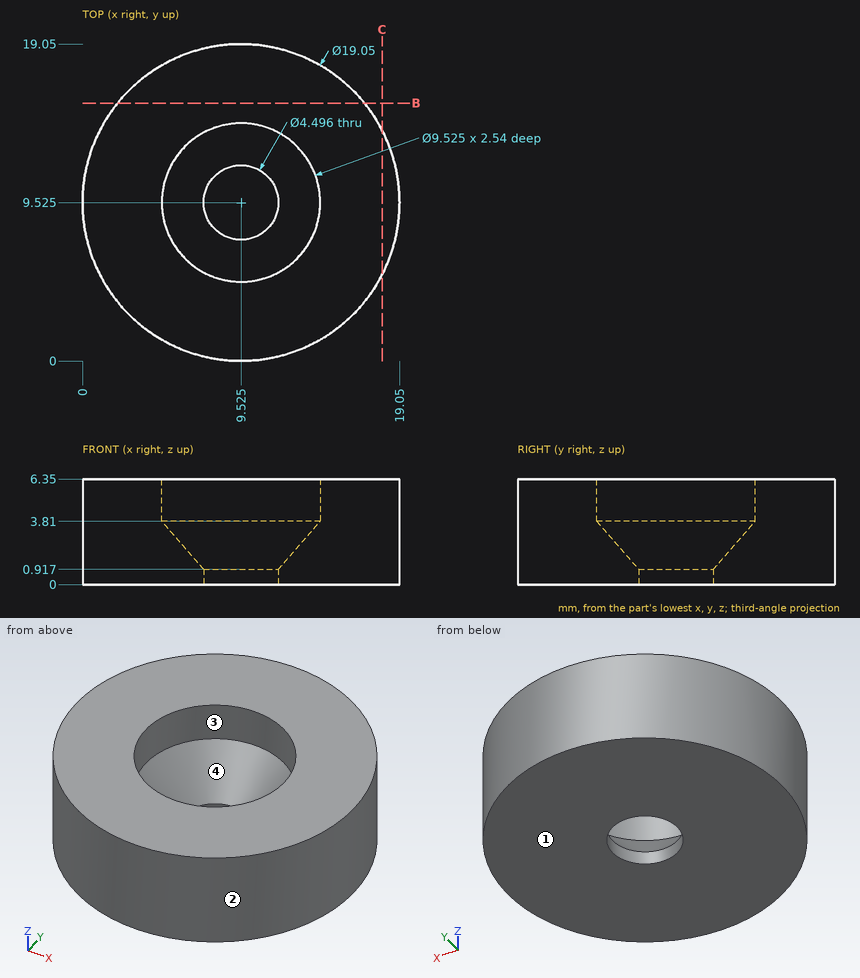
Answer from the drawing. Dimensions are ordinates in mm from the lowest x, y and z of the part. Coordinates: 2 decimals unless noted, no trailing zeros. Write each loop counter-clockwise with the first axis right and the second up, starting at its lowest first coordinate (ties: lowest second). Pieces come first, ordered by that corner, then holes. Notation, with made-up numbers: M 65.25,27 L 112.25,27 A21 ccw 112.25,33 Z; hole C 73,50.5 d2. An arc over 180 degrees is marked long. Write item = value, one per line.
1. Flat-ended cylindrical pins translate along their axes: pin 1 (3 mm diameter, centred on y = 4.5, z = 2.5, fed in from +X); pin 2 (8.5 mm diameter, centred on x = 9.525, y = 9.525, fed in from +Z); pin 3 (1.5 mm diameter, centred on y = 11, z = 1, fed in from -X). Find the tip coordinate at first contact, or state that the pin passes through.
Solution:
pin_1 = 18.37
pin_2 = 3.22
pin_3 = 0.03
2. The part is cut by section B-B (y = 15.5). Determine the outline of the cut face in (x, z), then the cut area to 3 significant figures.
Solution:
outline = M 2.11,0 L 16.94,0 L 16.94,6.35 L 2.11,6.35 Z
area = 94.2 mm2
3. The part is cut by section C-C (x = 18). Determine the outline of the cut face in (y, z), then the cut area to 3 significant figures.
Solution:
outline = M 5.18,0 L 13.87,0 L 13.87,6.35 L 5.18,6.35 Z
area = 55.2 mm2
4. Straight lines are drawn through the part: line 1 (Y direction, x = 10, z = 2); line 2 (Y direction, x = 10.75, z = 1.5); line 3 (X direction, y = 9.75, z = 5). For each, find the intervals that lie inside material, in ascending order. Write a range as from..to.
Solution:
line_1 = 0.01..6.37, 12.68..19.04
line_2 = 0.08..7.06, 11.99..18.97
line_3 = 0..4.77, 14.28..19.05
5. Determine the mould class of the marked faces 1, 2, 3 and 4 for opening direction X: released by +X, released by -X, zero draft, split by the parting line, or undercut.
Solution:
face_1 = zero draft
face_2 = split by the parting line
face_3 = undercut
face_4 = undercut
